Answer from the drawing. Dimensions are ordinates in mm from the lowest x, y and z of the part. A direction names the side the tool comes from. Round coordinates to 2 decimals unless told otherwise and drop trailing zeros. Loops run counter-clockwise (first coordinate to the right, second up) from the corner with the lowest first, then second, coordinate; pieces in that order, holes last. Notation, with made-up numbers: M 55.25,69.25 L 101.25,69.25 A25 ccw 101.25,84.25 Z; hole C 1,-21 d9. An arc over 180 degrees is marked long. Write each question's results on one line, items separated by ' | '.
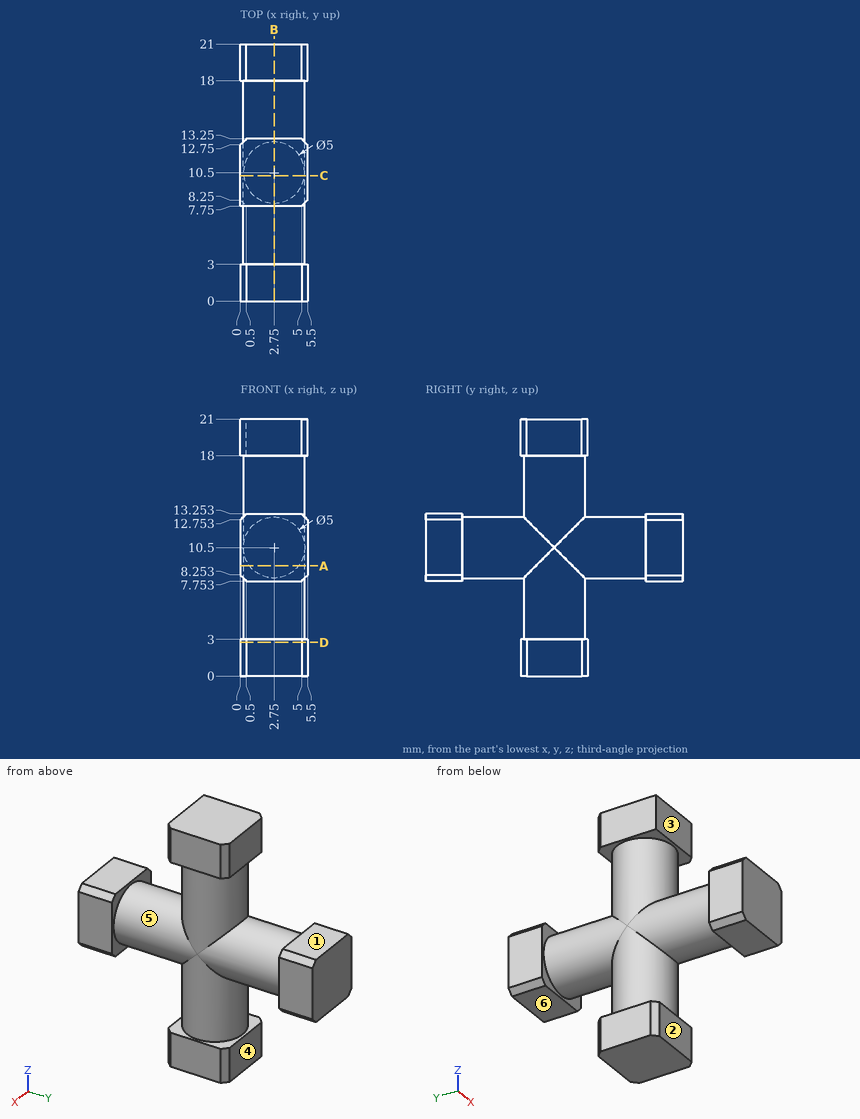
1. Given P1, Ø1.5, axis at x = 4, y = 3, coming from the +Z side; P2, Ø1.5, axis at y = 15.5, z = 8, coming from the -X side (1 decimal); P3, Ø0.9, axis at x = 2.5, z = 2, coming from the -Y side, each flat-ended and moving along its own axis, determine where each tip first touches the part or whether it passes through.
Completed:
P1: stops at z = 13.25 | P2: stops at x = 1 | P3: stops at y = 7.75
2. Find section A-A, the plane z = 9. Give the vertices of the cut face in (x, y).
Completed:
outline: M 0,0 L 5.5,0 L 5.5,3 L 4.75,3 L 4.75,9 A2.5 ccw 4.75,12 L 4.75,18 L 5.5,18 L 5.5,21 L 0,21 L 0,18 L 0.75,18 L 0.75,12 A2.5 ccw 0.75,9 L 0.75,3 L 0,3 Z
3. Find the intervals of material crossed by L1, parallel to Y at x = 2.75, z = 16.25; L2, parallel to Y at x = 0.45, z = 12.25; L3, parallel to Z at x = 1.7, y = 19.5, in increasing order.
Completed:
L1: y = 8 to 13 | L2: y = 0 to 3, 9.52 to 11.48, 18 to 21 | L3: z = 7.75 to 13.25
4. Find section B-B, the plane x = 2.75. Give the vertices of the cut face in (y, z).
Completed:
outline: M 0,7.75 L 3,7.75 L 3,8 L 8,8 L 8,3 L 7.75,3 L 7.75,0 L 13.25,0 L 13.25,3 L 13,3 L 13,8 L 18,8 L 18,7.75 L 21,7.75 L 21,13.25 L 18,13.25 L 18,13 L 13,13 L 13,18 L 13.25,18 L 13.25,21 L 7.75,21 L 7.75,18 L 8,18 L 8,13 L 3,13 L 3,13.25 L 0,13.25 Z
5. Which of the six approach directions +Z, -Z, +X, -X, +Y, -Y give full straight-line access (tool end or side, diameter ignored) to the marked faces 1, 2 and 3?
Completed:
face 1: +Z, +X, -X, +Y | face 2: -Z, +X, -X, -Y | face 3: +Z, +X, -X, -Y
6. Find section D-D, the plane z = 2.75. Give the vertices of the cut face in (x, y).
Completed:
outline: M 0,8.25 L 0.5,7.75 L 5,7.75 L 5.5,8.25 L 5.5,12.75 L 5,13.25 L 0.5,13.25 L 0,12.75 Z
7. Determine the mould class of the marked faces 4, 5 and 6 for opening direction Z: released by +Z, released by -Z, zero draft, split by the parting line, or undercut.
Completed:
face 4: zero draft | face 5: undercut | face 6: released by -Z
8. Find section C-C, the plane y = 10.25. Give the vertices of the cut face in (x, z), then the cut area to 3 significant figures.
Completed:
outline: M 0,0 L 5.5,0 L 5.5,3 L 5.24,3 L 5.24,10.25 A2.5 ccw 5.24,10.75 L 5.24,18 L 5.5,18 L 5.5,21 L 0,21 L 0,18 L 0.26,18 L 0.26,10.75 A2.5 ccw 0.26,10.25 L 0.26,3 L 0,3 Z | area: 108 mm2
